Design review of the part built by this model. Coordinates are the model's own, in mm. Give positions to 0.01 mm unless a question says otherwise; leave off trailing zeros. Loops run counter-clockwise (first coordinate to the right, second up) from the corner with the lowest first, then second, coordinate; pieces in that order, holes last.
from build123d import *

# Parameters (mm, degrees)
SKETCH1_R                    = 9.75
BOSS_EXTRUDE1_DEPTH          = 2
SKETCH2_R                    = 4
BOSS_EXTRUDE2_DEPTH          = 2.2
CHAMFER5_SIZE                = 0.2
CHAMFER6_SIZE                = 0.18
SKETCH8_R                    = 0.8
CUT_EXTRUDE1_DEPTH           = 14.962986787
CHAMFER7_SIZE                = 0.3
CIRPATTERN4_COUNT            = 8
CHAMFER7_OF_CIRPATTERN4_SIZE = 0.3


with BuildPart() as part:
    # Sketch1 → Boss-Extrude1 (new body)
    with BuildSketch(Plane.XY):
        Circle(SKETCH1_R)
    extrude(amount=BOSS_EXTRUDE1_DEPTH)

    # Sketch2 → Boss-Extrude2 (add)
    with BuildSketch(Plane.XY.offset(2)):
        Circle(SKETCH2_R)
    extrude(amount=BOSS_EXTRUDE2_DEPTH)

    # Chamfer5
    chamfer5_edges = [part.edges().sort_by_distance(p)[0] for p in [
        (-9.75, 0, 2),
    ]]
    chamfer(chamfer5_edges, length=CHAMFER5_SIZE)

    # Chamfer6
    chamfer6_edges = [part.edges().sort_by_distance(p)[0] for p in [
        (-4, 0, 4.2),
    ]]
    chamfer(chamfer6_edges, length=CHAMFER6_SIZE)

    # Sketch8 → Cut-Extrude1 (cut, through all)
    with BuildSketch(Plane.XY.offset(2)):
        with Locations((0, 8)):
            Circle(SKETCH8_R)
    cut_extrude1 = extrude(amount=-CUT_EXTRUDE1_DEPTH, mode=Mode.SUBTRACT)

    # Chamfer7
    chamfer7_edges = [part.edges().sort_by_distance(p)[0] for p in [
        (-0.8, 8, 2),
    ]]
    chamfer(chamfer7_edges, length=CHAMFER7_SIZE)

    # CirPattern4: Cut-Extrude1 ×8 about axis
    cirpattern4_axis = Axis((0, 0, 0), (0, 0, 1))
    for i in range(1, CIRPATTERN4_COUNT):
        add(cut_extrude1.rotate(cirpattern4_axis, i * 360 / CIRPATTERN4_COUNT), mode=Mode.SUBTRACT)

    # Chamfer7 of CirPattern4
    chamfer7_of_cirpattern4_edges = [part.edges().sort_by_distance(p)[0] for p in [
        (-6.222539674, 5.091168825, 2),
        (-8, -0.8, 2),
        (-5.091168825, -6.222539674, 2),
        (0.8, -8, 2),
        (6.222539674, -5.091168825, 2),
        (8, 0.8, 2),
        (5.091168825, 6.222539674, 2),
    ]]
    chamfer(chamfer7_of_cirpattern4_edges, length=CHAMFER7_OF_CIRPATTERN4_SIZE)


solid = part.part
Q1. Wall thickness on line 1 (Y direction, x = 0, z = 0.4); line 2 (Z direction, x = -3.5, y = 7); line 3 (X direction, y = 7.75, z = 1.9): over which ranges is each line inside the solid? List them lowest first.
Results:
line 1: y = -9.75 to -8.8, -7.2 to 7.2, 8.8 to 9.75
line 2: z = 0 to 2
line 3: x = -5.75 to -0.97, 0.97 to 5.75
Q2. Insertion check: pin 1 (2 mm diameter, centred on x = -8, y = 0, fed in from -Z); pin 2 (2 mm diameter, centred on x = 0, y = -8, fed in from +Z); pin 3 (2 mm diameter, centred on x = -5.5, z = 2.5, fed in from -Y); pin 4 (1.4 mm diameter, centred on x = 0, y = 8, fed in from -Z). Each pin has a flat end and moves straight along its axis. Give the tip position at first contact, or say it passes through.
Results:
pin 1: stops at z = 0
pin 2: stops at z = 1.9
pin 3: stops at y = -8.49
pin 4: passes through
Q3. Take a section at C-C (z = 0.35). Give the number of separate pieces and of enclosed holes in the cut face, plus the area to 3 significant figures.
Results:
separate pieces: 1
enclosed holes: 8
area: 283 mm2
Q4. Take a section at A-A (x = 0). Give the boundary of the cut face in (y, z), plus the area to 3 significant figures.
Results:
outline: (-9.75, 0) - (-8.8, 0) - (-8.8, 1.7) - (-9.1, 2) - (-9.55, 2) - (-9.75, 1.8) - close; (-7.2, 0) - (7.2, 0) - (7.2, 1.7) - (6.9, 2) - (4, 2) - (4, 4.02) - (3.82, 4.2) - (-3.82, 4.2) - (-4, 4.02) - (-4, 2) - (-6.9, 2) - (-7.2, 1.7) - close; (8.8, 0) - (9.75, 0) - (9.75, 1.8) - (9.55, 2) - (9.1, 2) - (8.8, 1.7) - close
area: 49.9 mm2
Q5. Draft analysis for pull direction X (two halves, no side actions). For faces 1 (the face through (4.9, -5.4, 0.9)), 2 (the face through (-0.867, -3.905, 2.996)), 3 (the face through (4, -2, 2)), state which applies: pulls with the +X half, pulls with the -X half, needs draft (parallel to the pull), parting line crosses it, or undercut.
Results:
face 1: undercut
face 2: parting line crosses it
face 3: needs draft
Q6. Take a section at D-D (z = 2.45). Give the boundary of the cut face in (x, y), plus the area to 3 significant figures.
Results:
outline: circle Ø8 at (0, 0)
area: 50.3 mm2
